Check sheet for the drawn part. Datum: minimum x, y, z corner. Units: mm. A direction names the side the tool comes from. Coordinates: 2 decimals unless noted, no trailing zeros. Order: outer loops, then holes, each group sorted by start corner. A loop starts at its lowest first (then second) coordinate and runs counter-clockwise, first axis right, second up.
1. Cross-section at B-B (x = 38.1). Enter the section's corners in (y, z), then the cut area to 3 significant figures.
2. Cross-section at A-A (z = 38.1). Enter the section's corners in (x, y), then the cut area to 3 significant figures.
3. Set-up check for the marked faces 5 and 6: record each of +Z, -Z, +X, -X, +Y, -Y from which the full face is reachable in a straight line by a thin tool's end or side.
4. Cross-section at C-C (y = 37.5). Enter the section's corners in (x, z).
5. Draft check along Z on the marked faces 1, 2, 3 and 4. Enter one of: released by +Z, released by -Z, zero draft, split by the parting line, or undercut.
6. Thickness scan on line 1 (Y direction, x = 24, z = 15.5); line 2 (Z direction, x = 54.5, y = 39.5); line 3 (Z direction, x = 38.1, y = 34). Record the ranges inside material, lowest first.
7. Cross-section at D-D (x = 66). Enter the section's corners in (y, z).
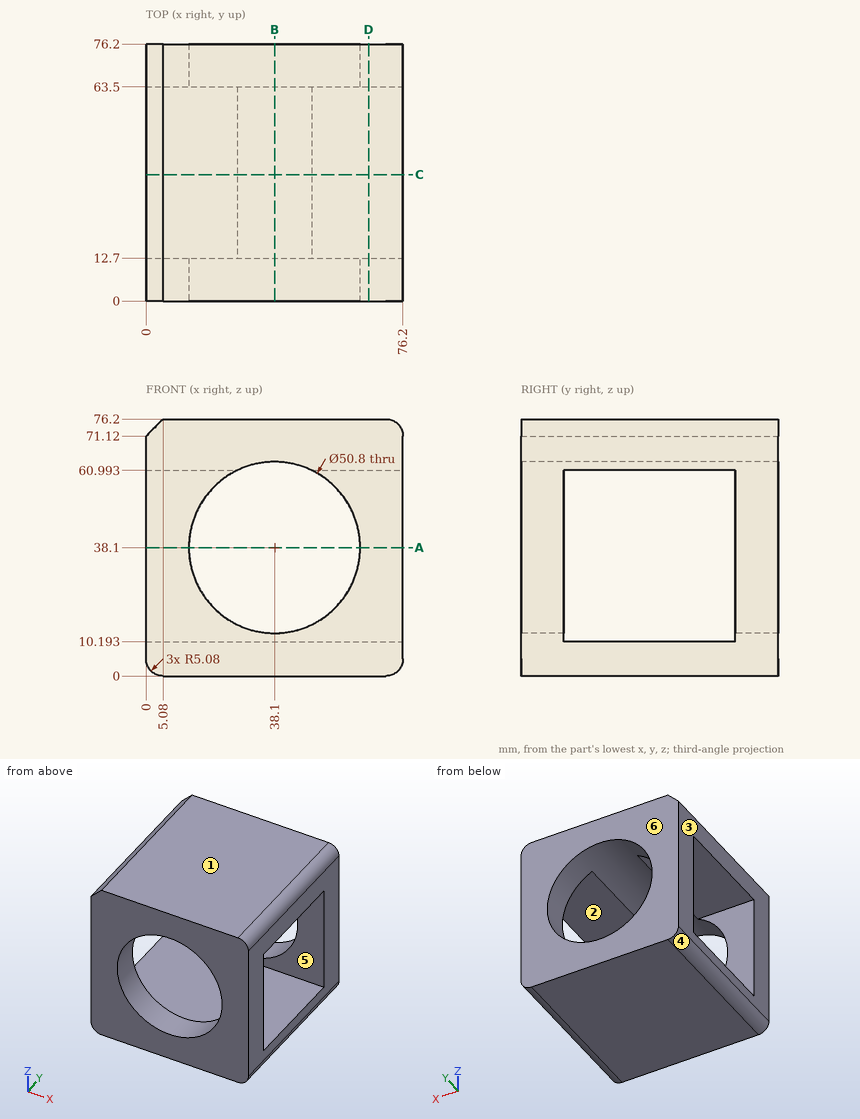
Data:
1. outline: (0, 0) - (76.2, 0) - (76.2, 12.7) - (63.5, 12.7) - (63.5, 10.19) - (12.7, 10.19) - (12.7, 12.7) - (0, 12.7) - close; (0, 63.5) - (76.2, 63.5) - (76.2, 76.2) - (0, 76.2) - close
1. area: 1,810 mm2
2. outline: (0, 0) - (12.7, 0) - (12.7, 12.7) - (0, 12.7) - close; (0, 63.5) - (12.7, 63.5) - (12.7, 76.2) - (0, 76.2) - close; (63.5, 0) - (76.2, 0) - (76.2, 12.7) - (63.5, 12.7) - close; (63.5, 63.5) - (76.2, 63.5) - (76.2, 76.2) - (63.5, 76.2) - close
2. area: 645 mm2
3. face 5: +X, -X
3. face 6: +Z, -Z, +X, -X, +Y
4. outline: (0, 5.08) arc R5.08 ccw to (5.08, 0) - (71.12, 0) arc R5.08 ccw to (76.2, 5.08) - (76.2, 10.19) - (0, 10.19) - close; (0, 60.99) - (27.1, 60.99) arc R25.4 cw to (49.1, 60.99) - (76.2, 60.99) - (76.2, 71.12) arc R5.08 ccw to (71.12, 76.2) - (5.08, 76.2) - (0, 71.12) - close
5. face 1: released by +Z
5. face 2: undercut
5. face 3: zero draft
5. face 4: released by -Z
6. line 1: y = 0 to 12.7, 63.5 to 76.2
6. line 2: z = 0 to 10.19, 60.99 to 76.2
6. line 3: z = 0 to 10.19, 63.5 to 76.2
7. outline: (0, 0) - (76.2, 0) - (76.2, 76.2) - (0, 76.2) - close; hole (12.7, 10.19) - (63.5, 10.19) - (63.5, 60.99) - (12.7, 60.99) - close
